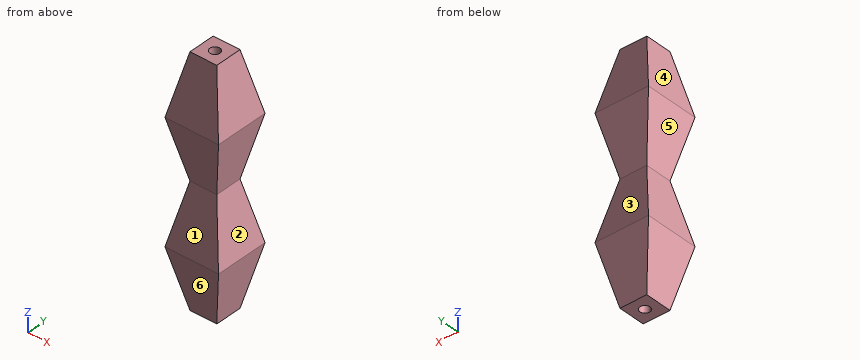
```python
from build123d import *

# Parameters (mm, degrees)
F0_W          = 101.6
F0_H          = 101.6
F1_DEPTH      = 457.2
F3_DEPTH      = 50.801
F3_DEPTH_BACK = 50.801
F5_DEPTH      = 50.801
F5_DEPTH_BACK = 50.801
F6_R          = 9.525
F7_DEPTH      = 457.201
F7_DEPTH_BACK = 708


# Not quite as in the source:
# - an extrude ends at something that could not be found from the text; its depth is read off the source's solid


with BuildPart() as f1:
    # F0 (on Top) → F1 (new body)
    with BuildSketch(Plane.XY):
        Rectangle(F0_W, F0_H)
    extrude(amount=F1_DEPTH)

    # F2 (on Front) → F3 (cut, two sides)
    with BuildSketch(Plane.XZ) as f3_sk:
        Polygon((-76.2, 0), (-50.8, 0), (-25.4, 0), (-50.8, 114.3), (-25.4, 228.6), (-50.8, 342.9), (-25.4, 457.2), (-50.8, 457.2), (-76.2, 457.2), align=None)
        Polygon((76.2, 457.2), (50.8, 457.2), (25.4, 457.2), (50.8, 342.9), (25.4, 228.6), (50.8, 114.3), (25.4, 0), (50.8, 0), (76.2, 0), align=None)
    extrude(amount=-F3_DEPTH, mode=Mode.SUBTRACT)
    extrude(f3_sk.sketch, amount=F3_DEPTH_BACK, mode=Mode.SUBTRACT)

    # F4 (on Right) → F5 (cut, two sides)
    with BuildSketch(Plane.YZ) as f5_sk:
        Polygon((76.2, 457.2), (50.8, 457.2), (25.4, 457.2), (50.8, 342.9), (25.4, 228.6), (50.8, 114.3), (25.4, 0), (50.8, 0), (76.2, 0), align=None)
        Polygon((-25.4, 457.2), (-50.8, 457.2), (-76.2, 457.2), (-76.2, 0), (-50.8, 0), (-25.4, 0), (-50.8, 114.3), (-25.4, 228.6), (-50.8, 342.9), align=None)
    extrude(amount=-F5_DEPTH, mode=Mode.SUBTRACT)
    extrude(f5_sk.sketch, amount=F5_DEPTH_BACK, mode=Mode.SUBTRACT)

    # F6 (on Top) → F7 (cut, two sides)
    with BuildSketch(Plane.XY) as f7_sk:
        Circle(F6_R)
    extrude(amount=F7_DEPTH, mode=Mode.SUBTRACT)
    extrude(f7_sk.sketch, amount=-F7_DEPTH_BACK, mode=Mode.SUBTRACT)


solid = f1.part
```
Input: part model. Units: mm. Frame: model coordinates. Face numbers are marked on the shaded views. A direction names the side the tool comes from. Give positions to 0.01 mm unless a question says otherwise; leave off trailing zeros. Loops run counter-clockwise (first coordinate to the right, second up) from the corner with the lowest first, then second, coordinate; pieces in that order, holes last.
1) Section query C-C on z = 328.5. Return the cut outline in (x, y) (3 decimals), and give its area (3 significant figures).
A:
outline: (-47.6, -47.6) - (47.6, -47.6) - (47.6, 47.6) - (-47.6, 47.6) - close; hole circle Ø19.05 at (0, 0)
area: 8,780 mm2
2) Contact query for flat-ended pins moving along their axis: pin 1 (5 mm diameter, centred on x = -23, z = 163.5, fed in from +Y); pin 2 (5 mm diameter, centred on y = -36.5, z = 332, fed in from +X); pin 3 (6 mm diameter, centred on x = -39.5, z = 284.5, fed in from +Y). Output: stop coordinate, or through.
A:
pin 1: stops at y = 40.42
pin 2: stops at x = 48.93
pin 3: stops at y = 38.45
3) Section query D-D on x = 0. Return the cut outline in (y, z) (3 decimals), and give its area (3 significant figures).
A:
outline: (-50.8, 114.3) - (-25.4, 0) - (-9.525, 0) - (-9.525, 457.2) - (-25.4, 457.2) - (-50.8, 342.9) - (-25.4, 228.6) - close; (9.525, 0) - (25.4, 0) - (50.8, 114.3) - (25.4, 228.6) - (50.8, 342.9) - (25.4, 457.2) - (9.525, 457.2) - close
area: 26,100 mm2
4) Line query: L1, parallel to Y at x = 0, z = 279.5 (3 decimals); L2, parallel to X at y = 0, z = 194.5 (3 decimals); L3, parallel to Y at x = -7.5, z = 39.5. Output: solid intervals per line, ascending.
A:
L1: y = -36.711 to -9.525, 9.525 to 36.711
L2: x = -32.978 to -9.525, 9.525 to 32.978
L3: y = -34.18 to -5.87, 5.87 to 34.18
5) Mould query, pull axis Z, two halves, no side actions, for the marked faces 4, 5 and 6. Classes: released by +Z, released by -Z, zero draft, split by the parting line, or undercut.
A:
face 4: released by +Z
face 5: undercut
face 6: released by -Z
6) Section query B-B on y = -40.5. Return the cut outline in (x, z).
A:
outline: (-50.8, 114.3) - (-40.5, 67.95) - (40.5, 67.95) - (50.8, 114.3) - (40.5, 160.65) - (-40.5, 160.65) - close; (-50.8, 342.9) - (-40.5, 296.55) - (40.5, 296.55) - (50.8, 342.9) - (40.5, 389.25) - (-40.5, 389.25) - close
7) Reachability of the marked faces 1, 2 and 3 from +Z, -Z, +X, -X, +Y, -Y: full face, straight path, thin tool, end or side. Return the list, or none.
A:
face 1: +X, -X, -Y
face 2: +X, +Y, -Y
face 3: +X, -X, +Y
8) Section query A-A on x = 32.5. Return the cut outline in (y, z).
A:
outline: (-50.8, 114.3) - (-32.5, 31.95) - (32.5, 31.95) - (50.8, 114.3) - (32.5, 196.65) - (-32.5, 196.65) - close; (-50.8, 342.9) - (-32.5, 260.55) - (32.5, 260.55) - (50.8, 342.9) - (32.5, 425.25) - (-32.5, 425.25) - close
